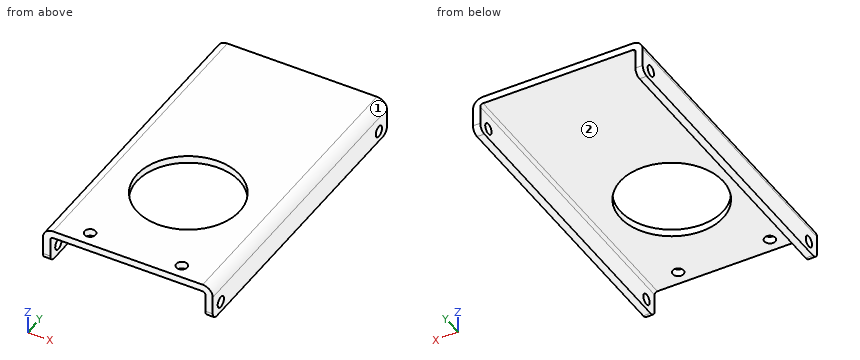
from build123d import *

# Parameters (mm, degrees)
SKETCH1_W                      = 76.3778
SKETCH1_H                      = 136.525
BASE_FLANGE1_DEPTH             = 3.2639
EDGE_FLANGE1_STRIP_W           = 15.5956
EDGE_FLANGE1_STRIP_H           = 3.2639
EDGE_FLANGE1_STRIP_CUT_DEPTH   = 136.525
EDGE_FLANGE1_STRIP_2_W         = 15.5956
EDGE_FLANGE1_STRIP_2_H         = 3.2639
EDGE_FLANGE1_STRIP_CUT_2_DEPTH = 136.525
EDGE_FLANGE1_DEPTH             = 136.525
EDGE_FLANGE1_BEND_DEPTH        = 136.525
F_10_0_1935_DIAMETER_HOLE1_D   = 4.9149
SKETCH32_R                     = 23.1775
CUT_EXTRUDE1_DEPTH             = 98.843921173
F_10_0_1935_DIAMETER_HOLE2_D   = 4.9149
FILLET1_R                      = 3.175


# Sheet-metal steps are written as plain solids
with BuildPart() as part:
    # Sketch1 → Base-Flange1 (new body)
    with BuildSketch(Plane.XY):
        with Locations((0, 20.933918)):
            Rectangle(SKETCH1_W, SKETCH1_H)
    extrude(amount=-BASE_FLANGE1_DEPTH)

    # Edge-Flange1 strip (across the edge) → Edge-Flange1 strip cut (cut)
    with BuildSketch(Plane(origin=(38.1889, 89.196418, -3.2639), x_dir=(-1, 0, 0), z_dir=(0, -1, 0))):
        with Locations((-3.2639, -1.63195)):
            Rectangle(EDGE_FLANGE1_STRIP_W, EDGE_FLANGE1_STRIP_H)
    extrude(amount=EDGE_FLANGE1_STRIP_CUT_DEPTH, mode=Mode.SUBTRACT)

    # Edge-Flange1 strip 2 (across the edge) → Edge-Flange1 strip cut 2 (cut)
    with BuildSketch(Plane(origin=(-38.1889, -47.328582, -3.2639), x_dir=(1, 0, 0), z_dir=(0, 1, 0))):
        with Locations((-3.2639, -1.63195)):
            Rectangle(EDGE_FLANGE1_STRIP_2_W, EDGE_FLANGE1_STRIP_2_H)
    extrude(amount=EDGE_FLANGE1_STRIP_CUT_2_DEPTH, mode=Mode.SUBTRACT)

    # Edge-Flange1 section (across the edge) → Edge-Flange1 (add)
    with BuildSketch(Plane(origin=(38.1889, 89.196418, -3.2639), x_dir=(-1, 0, 0), z_dir=(0, -1, 0))):
        with BuildLine():
            Line((0, 1.27), (0, 12.6111))
            Line((0, 12.6111), (3.2639, 12.6111))
            Line((3.2639, 12.6111), (3.2639, 1.27))
            ThreePointArc((3.2639, 1.27), (3.635874388, 0.371974388), (4.5339, 0))
            Line((4.5339, 0), (4.5339, -3.2639))
            ThreePointArc((4.5339, -3.2639), (1.327948565, -1.935951435), (0, 1.27))
        make_face()
    extrude(amount=EDGE_FLANGE1_DEPTH)

    # Edge-Flange1 section 2 (across the edge) → Edge-Flange1 bend (add)
    with BuildSketch(Plane(origin=(-38.1889, -47.328582, -3.2639), x_dir=(1, 0, 0), z_dir=(0, 1, 0))):
        with BuildLine():
            Line((0, 1.27), (0, 12.6111))
            Line((0, 12.6111), (3.2639, 12.6111))
            Line((3.2639, 12.6111), (3.2639, 1.27))
            ThreePointArc((3.2639, 1.27), (3.635874388, 0.371974388), (4.5339, 0))
            Line((4.5339, 0), (4.5339, -3.2639))
            ThreePointArc((4.5339, -3.2639), (1.327948565, -1.935951435), (0, 1.27))
        make_face()
    extrude(amount=EDGE_FLANGE1_BEND_DEPTH)

    # #10 (0.1935) Diameter Hole1 (through all)
    with Locations(Plane(origin=(38.1889, 0, 0), x_dir=(0, 0, -1), z_dir=(1, 0, 0))):
        with Locations((11.1125, 82.846418), (11.1125, -40.978582)):
            Hole(F_10_0_1935_DIAMETER_HOLE1_D / 2)

    # Sketch32 → Cut-Extrude1 (cut, through all)
    with BuildSketch(Plane(origin=(0, 0, -3.2639), x_dir=(-1, 0, 0), z_dir=(0, 0, -1))):
        Circle(SKETCH32_R)
    extrude(amount=-CUT_EXTRUDE1_DEPTH, mode=Mode.SUBTRACT)

    # #10 (0.1935) Diameter Hole2 (through all)
    with Locations(Plane.XY):
        with Locations((-20.6375, -40.978582), (20.6375, -40.978582)):
            Hole(F_10_0_1935_DIAMETER_HOLE2_D / 2)

    # Fillet1
    fillet1_edges = [part.edges().sort_by_distance(p)[0] for p in [
        (36.55695, 89.196418, -15.875),
        (36.55695, -47.328582, -15.875),
        (-36.55695, -47.328582, -15.875),
        (-36.55695, 89.196418, -15.875),
    ]]
    fillet(fillet1_edges, radius=FILLET1_R)


solid = part.part
CAD build for the part. Positions are in the model's coordinates, mm. Face numbers are marked on the shaded views. A direction names the side the tool comes from. Coordinates: 2 decimals unless noted, no trailing zeros. Loops run counter-clockwise (first coordinate to the right, second up) from the corner with the lowest first, then second, coordinate; pieces in that order, holes last. Notation, with made-up numbers: (44, 65.5) - (77, 65.5) arc R23 cw to (77, 87.5) - close; hole circle Ø7 at (75, 34). An arc over 180 degrees is marked (long way). Use one line per item in the form item = value. Start each with the question number.
1) Band-saw the part on D-D (x = -19.5). Give the cut face in (y, z).
2) Tool access for the marked faces 1 and 2: list every direction of +Z, -Z, +X, -X, +Y, -Y with a clear straight run to the whole face (end or side of a thin tool).
3) Band-saw the part on A-A (x = 0). Give the cut face in (y, z), and give its area (3 significant figures).
4) Band-saw the part on C-C (y = 53). Give the cut face in (x, z) (3 decimals), and give its area (3 significant figures).
5) Drill centre lines: L1, parallel to X at y = 44.5, z = -8 (3 decimals); L2, parallel to Z at x = 21, y = 81.5; L3, parallel to Y at x = 19, z = -1.5. Where is each one in solid material? Low to high. Write a range as from..to.
6) Band-saw the part on B-B (y = -5.5). Give the cut face in (x, z) (3 decimals), and give its area (3 significant figures).
7) Flat gauge pins, fed straight in: pin 1 (3 mm diameter, centred on x = -14, y = 35, fed in from +Z); pin 2 (4 mm diameter, centred on x = 26.5, y = -30, fed in from -Z); pin 3 (1.5 mm diameter, centred on x = 25, z = -5.5, fed in from +Y). Where does each tip first touch, or does it go through?
Check values:
q1.outline = (-47.33, -3.26) - (-43.16, -3.26) - (-43.16, 0) - (-47.33, 0) - close; (-38.8, -3.26) - (-12.53, -3.26) - (-12.53, 0) - (-38.8, 0) - close; (12.53, -3.26) - (89.2, -3.26) - (89.2, 0) - (12.53, 0) - close
q2.face_1 = +Z, +X, +Y, -Y
q2.face_2 = -Z, +Y, -Y
q3.outline = (-47.33, -3.26) - (-23.18, -3.26) - (-23.18, 0) - (-47.33, 0) - close; (23.18, -3.26) - (89.2, -3.26) - (89.2, 0) - (23.18, 0) - close
q3.area = 294 mm2
q4.outline = (-38.189, -15.875) - (-34.925, -15.875) - (-34.925, -4.534) arc R1.27 cw to (-33.655, -3.264) - (33.655, -3.264) arc R1.27 cw to (34.925, -4.534) - (34.925, -15.875) - (38.189, -15.875) - (38.189, -4.534) arc R4.534 ccw to (33.655, 0) - (-33.655, 0) arc R4.534 ccw to (-38.189, -4.534) - close
q4.area = 323 mm2
q5.L1 = -38.189..-34.925, 34.925..38.189
q5.L2 = -3.26..0
q5.L3 = -47.33..-42.81, -39.15..-13.27, 13.27..89.2
q6.outline = (-38.189, -15.875) - (-34.925, -15.875) - (-34.925, -4.534) arc R1.27 cw to (-33.655, -3.264) - (-22.515, -3.264) - (-22.515, 0) - (-33.655, 0) arc R4.534 ccw to (-38.189, -4.534) - close; (22.515, -3.264) - (33.655, -3.264) arc R1.27 cw to (34.925, -4.534) - (34.925, -15.875) - (38.189, -15.875) - (38.189, -4.534) arc R4.534 ccw to (33.655, 0) - (22.515, 0) - close
q6.area = 177 mm2
q7.pin_1 = 0
q7.pin_2 = -3.26
q7.pin_3 = through
